Build history of the part. All positions in model axes, mm. Round coordinates to 2 decimals unless told otherwise and drop trailing zeros. Write each loop counter-clockwise with the first axis right and the second up, starting at its lowest first coordinate (ties: lowest second). Pieces come first, ordered by that corner, then holes. Notation, with made-up numbers: (-37.75, -2) -> (-31.75, -2) arc R19 ccw to (-31.75, 20) -> close; hole circle Ø7 at (10, -39.5). An arc over 180 degrees is marked (long way). Answer as CSV lines item,"result".
from build123d import *

# Parameters (mm, degrees)
BASE_FLANGE1_DEPTH      = 50.8
CUT_EXTRUDE1_DEPTH      = 69.10802082
CUT_EXTRUDE1_DEPTH_BACK = 69.10802082
SKETCH6_W               = 25
SKETCH6_H               = 58.775055245


# Sheet-metal steps are written as plain solids
with BuildPart() as part:
    # Sketch1 → Base-Flange1 (new, symmetric)
    with BuildSketch(Plane(origin=(0, 0, 0), x_dir=(0, 0, -1), z_dir=(1, 0, 0))):
        with BuildLine():
            Line((45, -5.75), (0, -5.75))
            ThreePointArc((0, -5.75), (-2.786126343, 5.029910536), (4.874423043, -3.05))
            Line((4.874423043, -3.05), (2.755108676, -1.723913043))
            ThreePointArc((2.755108676, -1.723913043), (-1.574767064, 2.842992912), (0, -3.25))
            Line((0, -3.25), (45, -3.25))
            Line((45, -3.25), (45, -5.75))
        make_face()
    extrude(amount=BASE_FLANGE1_DEPTH, both=True)

    # Sketch6 → Cut-Extrude1 (cut, two sides: drawn at the far end of the back side and taken through both)
    with BuildSketch(Plane(origin=(0, 0, 0), x_dir=(1, 0, 0), z_dir=(0, 1, 0)).offset(-CUT_EXTRUDE1_DEPTH_BACK)):
        with Locations((-21.8, -21.887527623)):
            Rectangle(SKETCH6_W, SKETCH6_H)
        with Locations((21.8, -21.887527623)):
            Rectangle(SKETCH6_W, SKETCH6_H)
    extrude(amount=CUT_EXTRUDE1_DEPTH + CUT_EXTRUDE1_DEPTH_BACK, mode=Mode.SUBTRACT)


solid = part.part
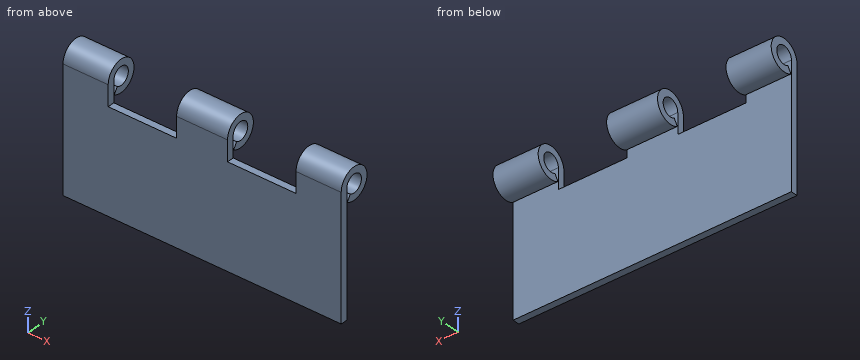
1. Cut at D-D, the plane x = 16. Write the cut outline in (y, z).
Results found:
outline,"(-5.75, -45) -> (-3.25, -45) -> (-3.25, -7.5) -> (-5.75, -7.5) -> close"
2. Cut at A-A, the plane y = 0. Write the cut outline in (x, z), then the cut area to 3 significant figures.
Results found:
outline,"(-50.8, -5.75) -> (-34.3, -5.75) -> (-34.3, -3.25) -> (-50.8, -3.25) -> close; (-50.8, 3.25) -> (-34.3, 3.25) -> (-34.3, 5.75) -> (-50.8, 5.75) -> close; (-9.3, -5.75) -> (9.3, -5.75) -> (9.3, -3.25) -> (-9.3, -3.25) -> close; (-9.3, 3.25) -> (9.3, 3.25) -> (9.3, 5.75) -> (-9.3, 5.75) -> close; (34.3, -5.75) -> (50.8, -5.75) -> (50.8, -3.25) -> (34.3, -3.25) -> close; (34.3, 3.25) -> (50.8, 3.25) -> (50.8, 5.75) -> (34.3, 5.75) -> close"
area,"258 mm2"
3. Probe line 1 along X through (y, z) = (5, 2); line 2 along Z through (x, y) = (-44.5, 0); line 3 along Y through (x, z) = (-37.5, -42). List the from-to ranges inside material, lowest first.
Results found:
line 1,"x = -50.8 to -34.3, -9.3 to 9.3, 34.3 to 50.8"
line 2,"z = -5.75 to -3.25, 3.25 to 5.75"
line 3,"y = -5.75 to -3.25"
4. Drop flat-ended pins along their axis: pin 1 Ø6 at (y, z) = (0, 0) entering from -X; pin 2 Ø2 at (x, y) = (18, -5) entering from +Z; pin 3 Ø13.5 at (x, z) = (-20.5, -30) entering from +Y; pin 4 Ø3 at (x, y) = (-8, -1.5) entering from -Z. Give the stop position or say it passes through.
Results found:
pin 1,"passes through"
pin 2,"stops at z = -7.5"
pin 3,"stops at y = -3.25"
pin 4,"stops at z = -5.75"
5. Cut at C-C, the plane z = -16.5. Write the cut outline in (x, y).
Results found:
outline,"(-50.8, -5.75) -> (50.8, -5.75) -> (50.8, -3.25) -> (-50.8, -3.25) -> close"
6. Cut at B-B, the plane x = 38.5. Write the cut outline in (y, z).
Results found:
outline,"(-5.75, -45) -> (-3.25, -45) -> (-3.25, 0) arc R3.25 cw (long way) to (-1.72, -2.76) -> (-3.05, -4.87) arc R5.75 ccw (long way) to (-5.75, 0) -> close"
